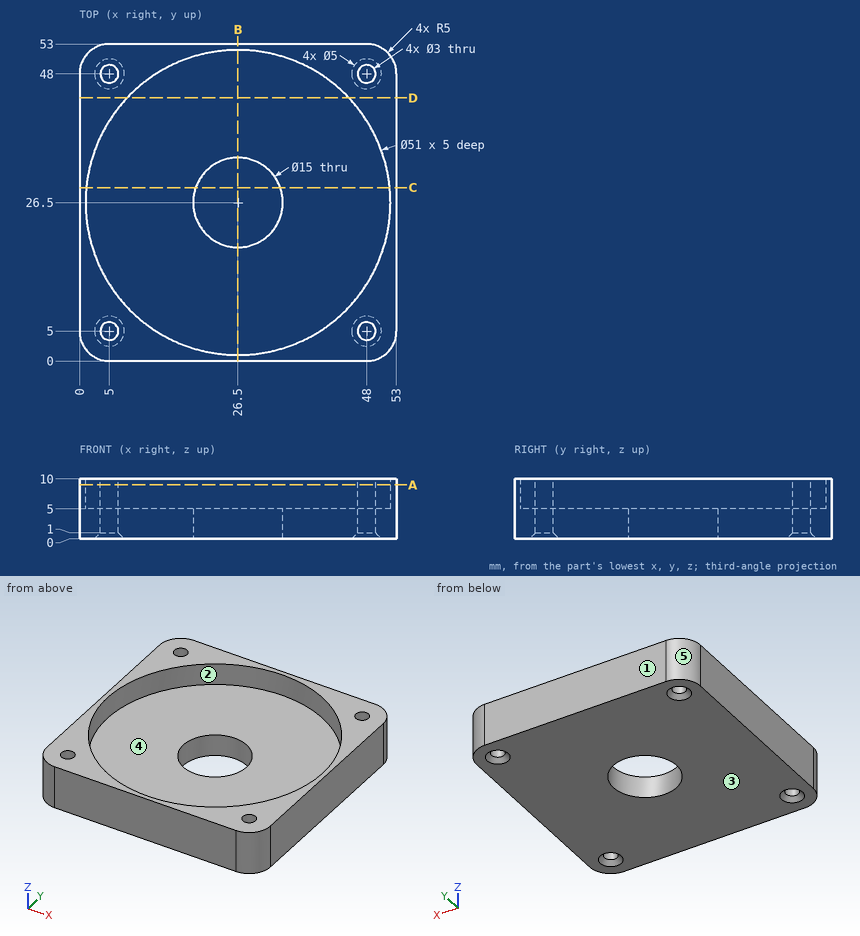
Print and shaded views of the part. All mm, measured from the part's lowest x, y and z. A direction names the side the tool comes from. Round coordinates to 2 decimals unless told otherwise and drop trailing zeros. Write each loop counter-clockwise with the first axis right and the second up, starting at its lowest first coordinate (ties: lowest second). Pieces come first, ordered by that corner, then holes. Notation, with made-up numbers: M 17,1.25 L 32,1.25 A27 ccw 32,23.25 Z; hole C 76,-30.75 d9. An arc over 180 degrees is marked long. One line per question, with ' | ' between items.
(1) Two-plate mould, pull along Y, no slides. Class the marked faces 1, 2 and 3: released by +Y, released by -Y, zero draft, split by the parting line, or undercut.
Answer key:
face 1: released by +Y | face 2: undercut | face 3: zero draft
(2) Saw through at A-A on z = 9. Write the cut outline in (x, y).
Answer key:
outline: M 0,5 A5 ccw 5,0 L 48,0 A5 ccw 53,5 L 53,48 A5 ccw 48,53 L 5,53 A5 ccw 0,48 Z; hole C 26.5,26.5 d51; hole C 5,5 d3; hole C 5,48 d3; hole C 48,5 d3; hole C 48,48 d3
(3) Pin check, flat tips, straight feed: pin 1 (4 mm diameter, centred on x = 28.5, y = 38, fed in from +Z); pin 2 (2.5 mm diameter, centred on x = 48, y = 5, fed in from +Z). Stop position of each tip, or through.
Answer key:
pin 1: stops at z = 5 | pin 2: passes through
(4) Probe line 1 along Y through (x, z) = (26.5, 1.65); line 2 along Y through (x, z) = (6, 4); line 3 along X through (y, z) = (6, 7). List the from-to ranges inside material, lowest first.
Answer key:
line 1: y = 0 to 19, 34 to 53 | line 2: y = 0 to 3.88, 6.12 to 46.88, 49.12 to 53 | line 3: x = 0 to 3.88, 6.12 to 11.33, 41.67 to 46.88, 49.12 to 53
(5) 3-axis set-ups, long thin cutter, end or side, ignore diameter. For the marked faces 4 and 5: which of +Z, -Z, +X, -X, +Y, -Y reach the whole face in a straight line?
Answer key:
face 4: +Z | face 5: +Z, -Z, -X, +Y
(6) Saw through at C-C on y = 29. Write the cut outline in (x, z), then the cut area to 3 significant figures.
Answer key:
outline: M 0,0 L 19.43,0 L 19.43,5 L 1.12,5 L 1.12,10 L 0,10 Z; M 33.57,0 L 53,0 L 53,10 L 51.88,10 L 51.88,5 L 33.57,5 Z | area: 206 mm^2
(7) Saw through at D-D on y = 44. Write the cut outline in (x, z).
Answer key:
outline: M 0,0 L 53,0 L 53,10 L 45.05,10 L 45.05,5 L 7.95,5 L 7.95,10 L 0,10 Z
(8) Saw through at B-B on x = 26.5. Write the cut outline in (y, z), then the cut area to 3 significant figures.
Answer key:
outline: M 0,0 L 19,0 L 19,5 L 1,5 L 1,10 L 0,10 Z; M 34,0 L 53,0 L 53,10 L 52,10 L 52,5 L 34,5 Z | area: 200 mm^2
